Work out the finished part from the listing and answer in its coordinate system (mm). A direction names the side the tool comes from. Coordinates: 2 decimals unless noted, no trailing zeros. Order: outer loops, then holes, each group sorted by start corner. A loop starts at its lowest first (then second) coordinate and runs counter-clockwise, first axis right, second up. Notation, with made-up numbers: M -20,48 L 11,48 A18 ccw 11,65 Z; hole C 38.25,33 d7. An arc over 180 degrees is marked long. Write item = value, one per line. Start each with the question number.
Q1. A tool of negligible diameter and unlimited length cuts with its end or side. For faces 1 (the flat face through (-15, -55, 98)), 2 (the cylindrical face through (-28.1, 48.72, -1.54)), 3 (the cylindrical face through (-2.131, 47.452, -1.54)), 4 (the flat face through (-35, 0, -2)), 5 (the flat face through (-30, 16, 52)), from which of +Z, -Z, +X, -X, +Y, -Y can it reach the whole face along a straight path? Write none if from no direction.
Q2. Find section D-D on z = -8.5. Give the vertices of the cut face in (x, y).
Q3. Find section C-C on x = -50.5. Give the vertices of the cut face in (y, z), and give its area (3 significant figures).
Q4. Straight lines are drawn through the part: line 1 along Z through (x, y) = (-47.5, 16); line 2 along Y through (x, z) = (-32, -38); line 3 along Z through (x, y) = (-29, -3.5). For each, find the intervals that lie inside material, in ascending order.
Q5. Each of these flat-tipped pins is pushed along its axis until it touches: P1, Ø1.5, axis at y = 5, z = -9.5, coming from the -X side; P2, Ø2, axis at y = -4.5, z = -59.5, coming from the +X side; P3, Ø1, axis at x = -15.5, z = 76, coming from the -Y side. Where does it stop, or does it pass through?
Q6. Find section A-A on z = 102. Give the number of separate pieces and of enclosed holes in the cut face, and give its area (3 significant figures).
```python
from build123d import *

# Parameters (mm, degrees)
BOSS_EXTRUDE1_DEPTH            = 110
BOSS_EXTRUDE3_START            = -109.99999999999999
BOSS_EXTRUDE3_DEPTH            = 10
SKETCH11_W                     = 7.99999999999995
SKETCH11_H                     = 7.7029575199640234
SKETCH11_H_2                   = 7.7029575199640306
CUT_EXTRUDE1_DEPTH             = 51.00000000000003
M4_CLEARANCE_HOLE1_D           = 4.5
M4_CLEARANCE_HOLE1_CSINK_D     = 4.55
M4_CLEARANCE_HOLE1_CSINK_ANGLE = 90
CUT_EXTRUDE2_START             = -19.999999999999996
SKETCH14_R                     = 20.000000000000004
CUT_EXTRUDE2_DEPTH             = 48
CUT_EXTRUDE3_DEPTH             = 2


# Read off the part's stored shape, not the designer's step: Mirror3
with BuildPart() as part:
    # Sketch1 → Boss-Extrude1 (new body)
    with BuildSketch(Plane.XY):
        with BuildLine():
            Line((-5.5e-16, 52.00000000000001), (-2, 52.00000000000001))
            Line((-2, 52.00000000000001), (-1.9999999999999996, 48.5))
            Line((-1.9999999999999996, 48.5), (-1.2e-16, 48.5))
            Line((-1.2e-16, 48.5), (0, 47.5))
            ThreePointArc((0, 47.5), (-2.1613294791041198, 47.45080246826976), (-4.318181818181816, 47.30331178453709))
            ThreePointArc((-4.318181818181816, 47.30331178453709), (-17.270978917519923, 40.87012512452316), (-22.499999999999996, 27.386127875258317))
            Line((-22.499999999999996, 27.386127875258317), (-22.499999999999996, -27.386127875258317))
            ThreePointArc((-22.499999999999996, -27.386127875258317), (-17.270978917519923, -40.870125124523156), (-4.318181818181816, -47.30331178453709))
            ThreePointArc((-4.318181818181816, -47.30331178453709), (-2.16132947910412, -47.45080246826977), (-1.16e-15, -47.5))
            Line((-1.16e-15, -47.5), (-1.27e-15, -48.49999999999999))
            Line((-1.27e-15, -48.49999999999999), (-2.0000000000000013, -48.49999999999999))
            Line((-2.0000000000000013, -48.49999999999999), (-2.000000000000001, -52))
            Line((-2.000000000000001, -52), (-9.8e-16, -52))
            Line((-9.8e-16, -52), (0, -60))
            ThreePointArc((0, -60), (-5.017575616780991, -59.789831367297616), (-9.999999999999995, -59.16079783099617))
            ThreePointArc((-9.999999999999995, -59.16079783099617), (-27.91287847477919, -48.945315646535164), (-34.99999999999999, -29.58039891549808))
            Line((-34.99999999999999, -29.58039891549808), (-34.99999999999999, 29.58039891549808))
            ThreePointArc((-34.99999999999999, 29.58039891549808), (-27.912878474779188, 48.945315646535164), (-9.999999999999995, 59.16079783099617))
            ThreePointArc((-9.999999999999995, 59.16079783099617), (-5.017575616780991, 59.78983136729761), (0, 60))
            Line((0, 60), (-5.5e-16, 52.00000000000001))
        make_face()
    extrude(amount=-BOSS_EXTRUDE1_DEPTH)

    # Sketch7 → Boss-Extrude3 (add)
    with BuildSketch(Plane.XY.offset(BOSS_EXTRUDE3_START)):
        with BuildLine():
            Line((0, 59.99999999999999), (0, -59.99999999999999))
            ThreePointArc((0, -59.99999999999999), (-59.99999999999999, 7.35e-15), (0, 59.99999999999999))
        make_face()
    extrude(amount=-BOSS_EXTRUDE3_DEPTH)

    # Sketch11 → Cut-Extrude1 (cut)
    with BuildSketch(Plane(origin=(-59.04024901745599, -4.1228e-13, 2.0975e-13), x_dir=(-3.55e-15, 6.98e-15, -1), z_dir=(-1, -6.98e-15, 3.55e-15))):
        with Locations((28.98410353274512, 56.148521240018084)):
            Rectangle(SKETCH11_W, SKETCH11_H)
        Polygon((98.00000000000352, 60.0000000000001), (106.0000000000035, 60.0000000000001), (106.0000000000035, 52.0000000000001), (98.0000000000035, 52.00000000000008), align=None)
        with Locations((28.98410353274512, -56.148521240016436)):
            Rectangle(SKETCH11_W, SKETCH11_H_2)
        Polygon((98.0000000000035, -51.99999999999843), (106.0000000000035, -51.99999999999845), (106.0000000000035, -59.99999999999845), (98.00000000000352, -59.99999999999845), align=None)
    extrude(amount=-CUT_EXTRUDE1_DEPTH, mode=Mode.SUBTRACT)

    # M4 Clearance Hole1 (through all)
    with Locations(Plane.ZY.offset(34.99999999999999)):
        with Locations((-28.984103533, -56.14852124), (-102, 56), (-28.984103533, 56.14852124), (-102, -56)):
            CounterSinkHole(M4_CLEARANCE_HOLE1_D / 2, M4_CLEARANCE_HOLE1_CSINK_D / 2, counter_sink_angle=M4_CLEARANCE_HOLE1_CSINK_ANGLE)

    # Sketch14 → Cut-Extrude2 (cut)
    with BuildSketch(Plane(origin=(0, 0, 0), x_dir=(0, 0, -1), z_dir=(1, 0, 0)).offset(CUT_EXTRUDE2_START)):
        with Locations((38.000000000000036, 0)):
            Circle(SKETCH14_R)
    extrude(amount=-CUT_EXTRUDE2_DEPTH, mode=Mode.SUBTRACT)

    # Sketch8 → Cut-Extrude3 (cut)
    with BuildSketch(Plane(origin=(0, 0, 0), x_dir=(0, 0, -1), z_dir=(1, 0, 0))):
        Polygon((117.00000000000003, 52.00000000000045), (117.0000000000004, -52.00000000000001), (110, -52), (110.00000000000074, -48.49999999999955), (113.50000000000074, -48.49999999999955), (113.50000000000007, 48.50000000000045), (110.0000000000014, 48.50000000000045), (110.00000000000004, 52.00000000000045), align=None)
    extrude(amount=-CUT_EXTRUDE3_DEPTH, mode=Mode.SUBTRACT)

    # Sketch22 → Cut-Revolve4 (revolve, cut)
    with BuildSketch(Plane.XY.offset(-38), mode=Mode.PRIVATE) as cut_revolve4_sk:
        Polygon((-34.99999999999999, -20.999999999999996), (-29.999999999999996, -20.999999999999996), (-30.000000000000004, -26.999999999999996), (-34.99999999999999, -26.999999999999996), align=None)
    revolve(cut_revolve4_sk.sketch.rotate(Axis((-1035, 3.47e-15, -38), (1, 0, 0)), 270), axis=Axis((-1035, 3.47e-15, -38), (1, 0, 0)), mode=Mode.SUBTRACT)

    # Mirror3: part across plane


with BuildPart() as part_1:
    add(part.part)
    add(part.part.mirror(Plane.XY))


solid = part_1.part
```
Findings below:
q1.face_1 = -X, -Y
q1.face_2 = -X, +Y
q1.face_3 = +X
q1.face_4 = -X, +Y, -Y
q1.face_5 = -X
q2.outline = M -35,-29.58 A30 ccw -10,-59.16 A60 ccw 0,-60 L 0,-52 L -2,-52 L -2,-48.5 L 0,-48.5 L 0,-47.5 A47.5 cw -4.32,-47.3 A20 cw -22.5,-27.39 L -22.5,27.39 A20 cw -4.32,47.3 A47.5 cw 0,47.5 L 0,48.5 L -2,48.5 L -2,52 L 0,52 L 0,60 A60 ccw -10,59.16 A30 ccw -35,29.58 Z
q3.outline = M -32.4,-120 L 32.4,-120 L 32.4,-110 L -32.4,-110 Z; M -32.4,110 L 32.4,110 L 32.4,120 L -32.4,120 Z
q3.area = 1,300 mm^2
q4.line_1 = -120 to -110, 110 to 120
q4.line_2 = -42.66 to -27, -21 to -20, 20 to 21, 27 to 42.66
q4.line_3 = -120 to -57.69, -18.31 to 18.31, 57.69 to 120
q5.P1 = -35
q5.P2 = -22.5
q5.P3 = -57.86
q6.separate_pieces = 3
q6.enclosed_holes = 0
q6.area = 1,580 mm^2
